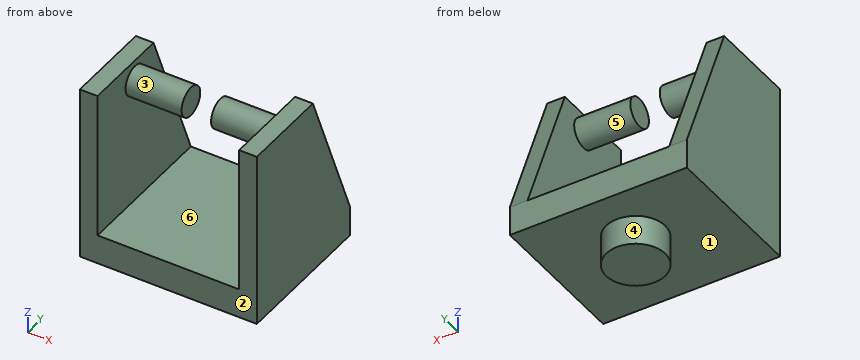
Autodesk Inventor part; units mm, degrees
ref_plane "YZ Plane" through (0, 0, 0) normal (1, 0, 0) x (0, 1, 0)
ref_plane "XZ Plane" through (0, 0, 0) normal (0, 1, 0) x (-1, 0, 0)
ref_plane "XY Plane" through (0, 0, 0) normal (0, 0, 1) x (1, 0, 0)
sketch "스케치1" plane through (0, 0, 0) normal (0, 0, 1) x (1, 0, 0)
  line L0 (15, -15) -> (-15, -15)
  line L1 (-15, -15) -> (-15, 15)
  line L2 (-15, 15) -> (15, 15)
  line L3 (15, 15) -> (15, -15)
  line L4 (15, -15) -> (-15, 15) construction
  line L5 (-15, -15) -> (15, 15) construction
  point P0 (0, 0)
  dimension "d0" = 30
  dimension "d1" = 30
extrude "돌출1" add sketch "스케치1" along normal blind 5
sketch "스케치2" plane through (0, 0, 5) normal (0, 0, 1) x (1, 0, 0)
  line L0 (-15, 15) -> (-15, -15)
  line L1 (-15, -15) -> (15, -15)
  line L2 (-15, 15) -> (-12, 15)
  line L3 (-12, 15) -> (-12, -15)
  line L4 (-12, -15) -> (-15, -15)
  line L5 (-15, -15) -> (-15, 15)
  line L6 (15, -15) -> (15, 15)
  line L7 (15, 15) -> (12, 15)
  line L8 (12, 15) -> (12, -15)
  line L9 (12, -15) -> (15, -15)
  line L10 (15, -15) -> (15, 15)
  point P0 (0, 0)
  dimension "d4" = 3
  dimension "d5" = 3
extrude "돌출2" add sketch "스케치2" along normal blind 30
sketch "스케치3" plane through (0, 0, 0) normal (0, 0, -1) x (-1, 0, 0)
  circle A0 centre (0, 0) radius 5
  dimension "d8" = 10
extrude "돌출3" add sketch "스케치3" along normal blind 5
sketch "스케치4" plane through (15, -15, 0) normal (1, 0, 0) x (0, 0, -1)
  line L0 (0, 0) -> (-39, 0)
  line L1 (-39, 0) -> (-26.5, 0)
  line L2 (-5, 0) -> (-35, 0)
  line L3 (-26.5, 0) -> (-26.5, 10)
  circle A0 centre (-26.5, 10) radius 2.5
  point P0 (0, 15)
  dimension "d11" = 39
  dimension "d12" = 12.5
  dimension "d13" = 5
  dimension "d14" = 10
extrude "돌출4" add sketch "스케치4" against normal blind 12.5
sketch "스케치5" plane through (-15, -15, 0) normal (-1, 0, 0) x (0, 0, 1)
  circle A0 centre (26.5, 10) radius 2.5
  point P0 (0, 15)
extrude "돌출5" add sketch "스케치5" against normal blind 12.5
sketch "스케치6" plane through (15, -15, 0) normal (1, 0, 0) x (0, 0, -1)
  line L0 (0, 30) -> (-35, 30)
  line L1 (-5, 30) -> (-35, 30)
  line L2 (-5, 30) -> (-35, 30)
  line L3 (0, 30) -> (-35, 30)
  line L4 (-5, 0) -> (-5, 30)
  line L5 (-5, 30) -> (-5, 0)
  line L6 (0, 30) -> (-35, 30)
  line L7 (-5, 30) -> (-5, 0)
  line L8 (0, 30) -> (-5, 30)
  line L9 (-5, 30) -> (-10, 30)
  line L10 (-5, 30) -> (-35, 30)
  line L11 (-35, 0) -> (-35, 30)
  line L12 (-10, 30) -> (-35, 30)
  line L13 (-35, 30) -> (-35, 20)
  line L14 (-35, 20) -> (-10, 30)
  circle A0 centre (-26.5, 10) radius 2.5
  line L15 (0, 0) -> (-35, 0)
  line L16 (-35, 0) -> (-30, 0)
  line L17 (-30, 0) -> (-30, 22)
  point P0 (0, 15)
  dimension "d19" = 5
  dimension "d20" = 5
  dimension "d21" = 10
  dimension "d22" = 5
extrude "돌출6" cut sketch "스케치6" against normal through all contours L14 L11 L0 | L17 L15 L11 L14
sketch "스케치7" plane through (15, -15, 0) normal (1, 0, 0) x (0, 0, -1)
  line L0 (-5, 0) -> (-5, 30)
  line L1 (-5, 30) -> (-5, 25)
  line L2 (-5, 30) -> (-5, 0)
  line L3 (-5, 25) -> (-30, 25)
  line L4 (-30, 22) -> (-30, 0)
  circle A0 centre (-26.5, 10) radius 2.5
  line L5 (-30, 25) -> (-30, 15)
  line L6 (-30, 15) -> (-5, 25)
  line L7 (-30, 22) -> (-30, 0)
  line L8 (0, 0) -> (-30, 0)
  line L9 (0, 0) -> (0, 30)
  line L10 (0, 30) -> (-10, 30)
  line L11 (-10, 30) -> (-30, 22)
  point P0 (0, 15)
  dimension "d25" = 5
  dimension "d26" = 10
extrude "돌출7" cut sketch "스케치7" against normal through all contours L3 L11 L10 L0 | L6 L4 L11 L3
sketch "스케치8" plane through (15, -15, 0) normal (1, 0, 0) x (0, 0, -1)
  line L0 (0, 0) -> (0, 30)
  line L1 (0, 30) -> (0, 25)
  line L2 (0, 25) -> (-5, 25)
  line L3 (0, 30) -> (-5, 30)
  line L4 (-5, 25) -> (-5, 30)
  line L5 (0, 30) -> (-5, 30)
  point P0 (0, 15)
  dimension "d29" = 5
extrude "돌출8" cut sketch "스케치8" against normal through all
properties part number "castor_link" material "알루미늄 6061"
For this review, take the finished solid that the model builds, in its own axes (mm). Face numbers are marked on the shaded views. A direction names the side the tool comes from. Give positions to 0.01 mm unless a question says otherwise; leave off trailing zeros. Loops run counter-clockwise (first coordinate to the right, second up) from the corner with the lowest first, then second, coordinate; pieces in that order, holes last. Notation, with made-up numbers: M 42.5,-28.75 L 55.5,-28.75 A15 ccw 55.5,-24.75 Z; hole C 34,41 d5. An arc over 180 degrees is marked long. Answer as a JSON object with one key per item and string values. Group by question number.
Q1. Add section D-D on x = 0. Give the boundary of the cut face in (y, z).
Q2. For probe 1 along X at (y, z) = (0.25, 7.5); probe 2 along Z at (x, y) = (11.25, -9.25); probe 3 along Z at (x, y) = (-6.75, -5.25), list the stretches that pass through material, from the lowest coordinate up. Write a range as [from, to].
Q3. Insertion check: P1, Ø8, axis at x = 9.5, y = -2, coming from the -Z side; P2, Ø8, axis at x = -0.5, y = 6.5, coming from the -Z side. Each pin has a flat end and moves straight along its axis. Give the tip position at first contact, or say it passes through.
Q4. Tool access review of the marked faces 4, 5 and 6: name each direction out of +Z, -Z, +X, -X, +Y, -Y from which nothing blocks a thin tool from reaching the whole face with its end or side.
Q5. Add section B-B on x = -4. Give the boundary of the cut face in (y, z).
Q6. Add section C-C on y = 6. Give the boundary of the cut face in (x, z).
Q7. Mouldability with a two-part tool opening along Z and no side actions: class the marked faces 1, 2 and 3 as +Z half, -Z half, draft (parallel to the pull), parting line (faces both ways), or undercut.
Q8. Add section A-A on z = 8.5. Give the boundary of the cut face in (x, y), and give its area (3 significant figures).
Checked values:
{
 "1": {"outline": "M -15,0 L -5,0 L -5,-5 L 5,-5 L 5,0 L 10,0 L 10,5 L -15,5 Z"},
 "2": {"probe 1": "[-15, -12], [12, 15]", "probe 2": "[0, 5]", "probe 3": "[0, 5], [24.01, 28.99]"},
 "3": {"P1": "z = 0", "P2": "z = -5"},
 "4": {"face 4": "-Z", "face 5": "none", "face 6": "+Y, -Y"},
 "5": {"outline": "M -15,0 L -3,0 L -3,-5 L 3,-5 L 3,0 L 10,0 L 10,5 L -15,5 Z; C -5,26.5 d5"},
 "6": {"outline": "M -15,0 L 15,0 L 15,15 L 12,15 L 12,5 L -12,5 L -12,15 L -15,15 Z"},
 "7": {"face 1": "-Z half", "face 2": "draft", "face 3": "undercut"},
 "8": {"outline": "M -15,-15 L -12,-15 L -12,8.6 L -15,8.6 Z; M 12,-15 L 15,-15 L 15,8.6 L 12,8.6 Z", "area": "142 mm²"}
}
